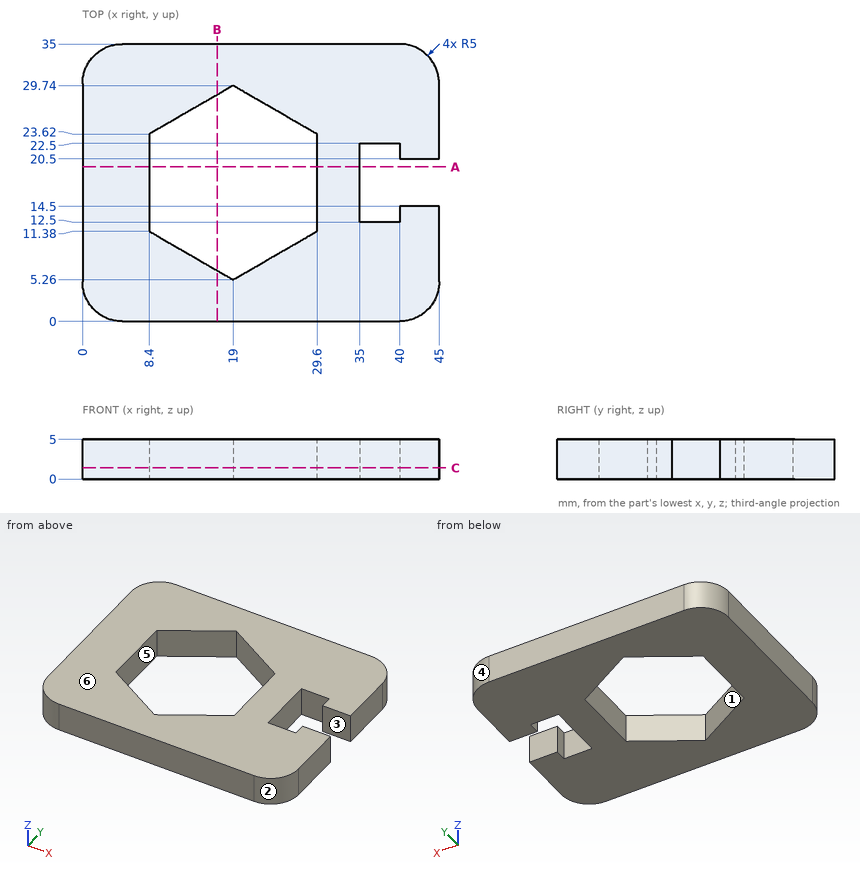
Verification items for this drawing (mm, ordinates from the low corner). A direction names the side the tool comes from. Round coordinates to 2 decimals unless told otherwise and drop trailing zeros. Loops run counter-clockwise (first coordinate to the right, second up) from the corner with the lowest first, then second, coordinate; pieces in that order, holes last. Notation, with made-up numbers: (60.25, 60.25) - (104.25, 60.25) arc R25 ccw to (104.25, 74.25) - close; hole circle Ø2 at (32, 63). An arc over 180 degrees is marked (long way). Answer as CSV lines item,"result". Start each with the question number.
Item 1: Depth check by flat-ended pin: P1, Ø0.6, axis at y = 21.5, z = 1.5, coming from the -X side; P2, Ø1.5, axis at x = 43.5, z = 3.5, coming from the -Y side; P3, Ø2, axis at x = 25, y = 12, coming from the -Z side; P4, Ø2.5, axis at x = 42, z = 2, coming from the +Y side. Enter the tip coordinate at first touch or a pass-through.
Item 2: Set-up check for the marked faces 1, 2 and 3: record each of +Z, -Z, +X, -X, +Y, -Y from which the full face is reachable in a straight line by a thin tool's end or side.
Item 3: Scan lines: line 1 (X direction, y = 13.5, z = 2.65); line 2 (X direction, y = 23.5, z = 4.1); line 3 (Y direction, x = 19, z = 4.8). Record each from-to range of solid material in increasing order. Write a range as [from, to].
Item 4: Release check for a two-part mould opening along X. For the marked faces 4, 5 and 6 record: +X half, -X half, draft (parallel to the pull), parting line (faces both ways), or undercut.
Item 5: Section check A-A (y = 19.5). Record the boundary of the cut face in (x, z).
Item 6: Section check C-C (z = 1.4). Record the boundary of the cut face in (x, y), and give its area (3 significant figures).
Item 7: Section check B-B (x = 17). Record the boundary of the cut face in (y, z) (3 decimals).
Report:
1,P1,"stops at x = 0"
1,P2,"stops at y = 0.82"
1,P3,"passes through"
1,P4,"stops at y = 34.94"
2,face 1,"+Z, -Z"
2,face 2,"+Z, -Z, +X, -Y"
2,face 3,"+Z, -Z, +X"
3,line 1,"x = [0, 8.4], [29.6, 35], [40, 45]"
3,line 2,"x = [0, 8.4], [29.6, 45]"
3,line 3,"y = [0, 5.26], [29.74, 35]"
4,face 4,"+X half"
4,face 5,"undercut"
4,face 6,"draft"
5,outline,"(0, 0) - (8.4, 0) - (8.4, 5) - (0, 5) - close; (29.6, 0) - (35, 0) - (35, 5) - (29.6, 5) - close"
6,outline,"(0, 5) arc R5 ccw to (5, 0) - (40, 0) arc R5 ccw to (45, 5) - (45, 14.5) - (40, 14.5) - (40, 12.5) - (35, 12.5) - (35, 22.5) - (40, 22.5) - (40, 20.5) - (45, 20.5) - (45, 30) arc R5 ccw to (40, 35) - (5, 35) arc R5 ccw to (0, 30) - close; hole (8.4, 11.38) - (19, 5.26) - (29.6, 11.38) - (29.6, 23.62) - (19, 29.74) - (8.4, 23.62) - close"
6,area,"1,080 mm2"
7,outline,"(0, 0) - (6.415, 0) - (6.415, 5) - (0, 5) - close; (28.585, 0) - (35, 0) - (35, 5) - (28.585, 5) - close"
